The model under review builds one solid part; all positions refer to its coordinate system, in mm. Face numbers are marked on the shaded views. Coordinates: 2 decimals unless noted, no trailing zeros. Write each loop counter-clockwise with the first axis right and the second up, starting at its lowest first coordinate (ties: lowest second). Pieces come first, ordered by that corner, then holes.
1) For line 1 (X direction, y = 59.5, z = 0); line 2 (Z direction, x = 71.5, y = 112); line 3 (X direction, y = 105.5, z = -16.5), list the stretches that pass through material, from the lowest coordinate up.
2) Add section C-C, the plane y = 173.5. State the section outline as (x, z) points.
3) Add section B-B, the plane x = 0. State the section outline as (y, z) points.
4) For P1, Ø3, axis at x = 63, z = -24.5, coming from the -Y side; P2, Ø12, axis at y = 30.5, z = -34, coming from the +X side; P3, Ø2, axis at y = 107, z = -70, coming from the +X side, all flat-tipped, find the tip position at first contact; note any pin that passes through.
5) Mouldability with a two-part tool opening along Z and no side actions: class the marked faces 1 and 2 as released by +Z, released by -Z, zero draft, split by the parting line, or undercut.
6) Add section A-A, the plane z = 0. State the section outline as (x, y) points.
from build123d import *

# Parameters (mm, degrees)
SKETCH1_R           = 86.36
SKETCH1_R_2         = 80.518
BOSS_EXTRUDE1_DEPTH = 5.08
SKETCH2_R           = 95.758
BOSS_EXTRUDE2_DEPTH = 5.08
SKETCH3_R           = 95.758
SKETCH3_R_2         = 90.678
BOSS_EXTRUDE3_DEPTH = 175.26
FILLET1_R           = 6.35


with BuildPart() as part:
    # Sketch1 → Boss-Extrude1 (new body)
    with BuildSketch(Plane(origin=(0, 0, 0), x_dir=(1, 0, 0), z_dir=(0, 1, 0))):
        with Locations(Location((0, 0, 0), (0, 0, 270))):
            Circle(SKETCH1_R)
        with Locations(Location((0, 0, 0), (0, 0, 270))):
            Circle(SKETCH1_R_2, mode=Mode.SUBTRACT)
    extrude(amount=BOSS_EXTRUDE1_DEPTH)

    # Sketch2 → Boss-Extrude2 (add)
    with BuildSketch(Plane(origin=(0, 5.08, 0), x_dir=(1, 0, 0), z_dir=(0, 1, 0))):
        with Locations(Location((0, 0, 0), (0, 0, 270))):
            Circle(SKETCH2_R)
    extrude(amount=BOSS_EXTRUDE2_DEPTH)

    # Sketch3 → Boss-Extrude3 (add)
    with BuildSketch(Plane(origin=(0, 10.16, 0), x_dir=(1, 0, 0), z_dir=(0, 1, 0))):
        with Locations(Location((0, 0, 0), (0, 0, 270))):
            Circle(SKETCH3_R)
        with Locations(Location((0, 0, 0), (0, 0, 270))):
            Circle(SKETCH3_R_2, mode=Mode.SUBTRACT)
    extrude(amount=BOSS_EXTRUDE3_DEPTH)

    # Fillet1
    fillet1_edges = [part.edges().sort_by_distance(p)[0] for p in [
        (0, 10.16, -90.678),
        (0, 5.08, -95.758),
    ]]
    fillet(fillet1_edges, radius=FILLET1_R)


solid = part.part
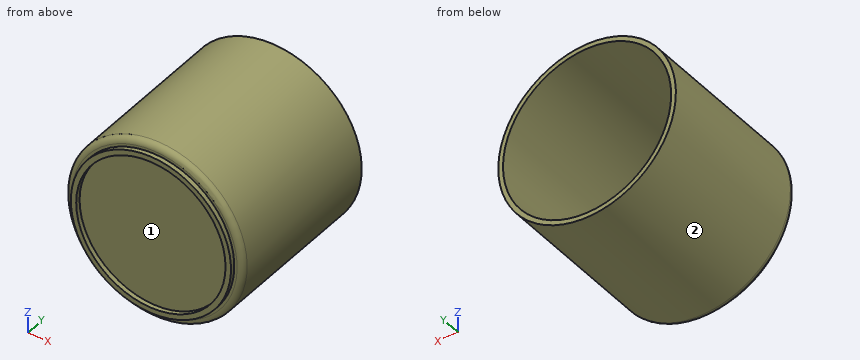
Geometry results:
1. line 1: x = -95.76 to -90.68, 90.68 to 95.76
1. line 2: z = -63.7 to -55.77, 55.77 to 63.7
1. line 3: x = -94.33 to -89.16, 89.16 to 94.33
2. outline: circle Ø191.52 at (0, 0); hole circle Ø181.36 at (0, 0)
3. outline: (0, -86.36) - (5.08, -86.36) - (5.08, -89.41) arc R6.35 ccw to (11.43, -95.76) - (185.42, -95.76) - (185.42, -90.68) - (16.51, -90.68) arc R6.35 cw to (10.16, -84.33) - (10.16, 84.33) arc R6.35 cw to (16.51, 90.68) - (185.42, 90.68) - (185.42, 95.76) - (11.43, 95.76) arc R6.35 ccw to (5.08, 89.41) - (5.08, 86.36) - (0, 86.36) - (0, 80.52) - (5.08, 80.52) - (5.08, -80.52) - (0, -80.52) - close
4. P1: stops at y = 5.08
4. P2: stops at x = 91.57
4. P3: stops at x = 66.4
5. face 1: undercut
5. face 2: split by the parting line
6. outline: (-95.76, 11.43) arc R6.35 ccw to (-89.41, 5.08) - (-86.36, 5.08) - (-86.36, 0) - (-80.52, 0) - (-80.52, 5.08) - (80.52, 5.08) - (80.52, 0) - (86.36, 0) - (86.36, 5.08) - (89.41, 5.08) arc R6.35 ccw to (95.76, 11.43) - (95.76, 185.42) - (90.68, 185.42) - (90.68, 16.51) arc R6.35 cw to (84.33, 10.16) - (-84.33, 10.16) arc R6.35 cw to (-90.68, 16.51) - (-90.68, 185.42) - (-95.76, 185.42) - close
